Geometry check sheet. Reference: drawing and pictorial views, mm from the part's lowest x, y, z. Give positions to 0.01 mm unless a question says otherwise; leave off trailing zeros. Write each loop counter-clockwise with the first axis right and the second up, starting at its lowest first coordinate (ties: lowest second). Pieces come first, ordered by that corner, then holes. Notation, with made-up numbers: (57, -19.5) -> (99, -19.5) arc R7 ccw to (99, -12.5) -> close; hole circle Ø8 at (58.5, 17). An arc over 180 degrees is marked (long way). Use a Markdown table: item, result. Add a question column.
1. Scan lines: probe 1 along Y at (x, z) = (84, 2.7); probe 2 along X at (y, z) = (39, 2) (1 decimal); probe 3 along X at (y, z) = (73, 4.6) (1 decimal). Record each from-to range of solid material in increasing order. Write a range as [from, to].
2. Cross-section at C-C (z = 2.35). Enter the section's corners in (x, y), then the cut area to 3 significant figures.
3. Gauge pin test, flat ends, axial feed: P1, Ø1, axis at y = 96.5, z = 3, coming from the -X side (1 decimal); P2, Ø1.8, axis at y = 116, z = 2, coming from the -X side; P3, Ø6.5, axis at x = 84, y = 70.77, coming from the +Z side. Record the tip position at first contact, or that the pin passes through.
4. Cross-section at A-A (y = 40). Enter the section's corners in (x, z).
5. Cross-section at B-B (x = 84). Enter the section's corners in (y, z).
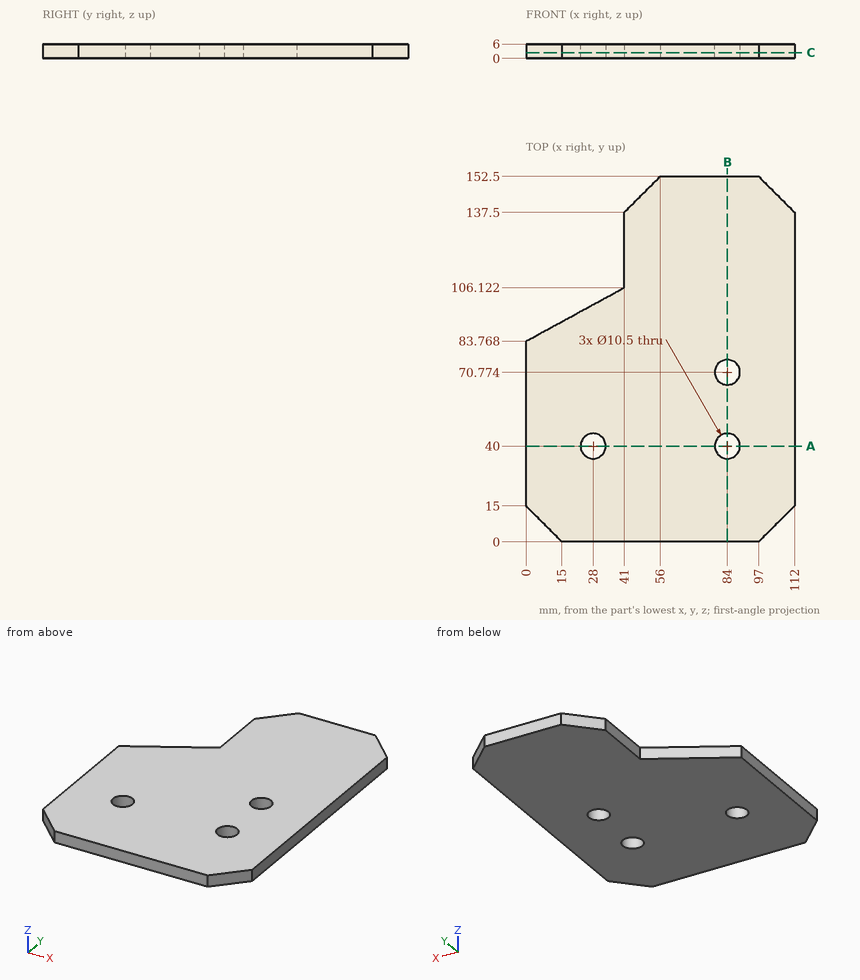
Worked answers:
| question | item | result |
|---|---|---|
| 1 | probe 1 | y = [0, 34.75], [45.25, 65.52], [76.02, 152.5] |
| 1 | probe 2 | x = [0, 22.8], [33.2, 78.8], [89.2, 112] |
| 1 | probe 3 | x = [0, 79.2], [88.8, 112] |
| 2 | outline | (0, 15) -> (15, 0) -> (97, 0) -> (112, 15) -> (112, 137.5) -> (97, 152.5) -> (56, 152.5) -> (41, 137.5) -> (41, 106.12) -> (0, 83.77) -> close; hole circle Ø10.5 at (28, 40); hole circle Ø10.5 at (84, 40); hole circle Ø10.5 at (84, 70.77) |
| 2 | area | 14,000 mm² |
| 3 | P1 | stops at x = 22.4 |
| 3 | P2 | stops at x = 41 |
| 3 | P3 | passes through |
| 4 | outline | (0, 0) -> (22.75, 0) -> (22.75, 6) -> (0, 6) -> close; (33.25, 0) -> (78.75, 0) -> (78.75, 6) -> (33.25, 6) -> close; (89.25, 0) -> (112, 0) -> (112, 6) -> (89.25, 6) -> close |
| 5 | outline | (0, 0) -> (34.75, 0) -> (34.75, 6) -> (0, 6) -> close; (45.25, 0) -> (65.52, 0) -> (65.52, 6) -> (45.25, 6) -> close; (76.02, 0) -> (152.5, 0) -> (152.5, 6) -> (76.02, 6) -> close |
